For this review, take the finished solid that the model builds, in its own axes (mm). Round coordinates to 2 decimals unless told otherwise and drop trailing zeros. Write each loop counter-clockwise with the first axis right and the second up, starting at its lowest first coordinate (ties: lowest second). Pieces come first, ordered by that corner, then holes.
Autodesk Inventor part; units mm, degrees
ref_plane "YZ Plane" through (0, 0, 0) normal (1, 0, 0) x (0, 1, 0)
ref_plane "XZ Plane" through (0, 0, 0) normal (0, 1, 0) x (-1, 0, 0)
ref_plane "XY Plane" through (0, 0, 0) normal (0, 0, 1) x (1, 0, 0)
sketch "Sketch1" plane through (0, 0, 0) normal (0, 1, 0) x (-1, 0, 0)
  line L0 (0.3129, 0) -> (0.3129, 5)
  line L1 (3.3129, 5) -> (3.3129, 0)
  arc A0 (3.3129, 5) -> (0.3129, 5) centre (1.8129, 5) ccw
  arc A1 (0.3129, 0) -> (3.3129, 0) centre (1.8129, 0) ccw
  point P0 (0, 0)
  dimension "d1" = 5
  dimension "d7" = 3
extrude "Extrusion1" add sketch "Sketch1" along normal blind 3
chamfer "Chamfer1" distance 0.2 angle 45 8 edges at (-0.3129, 3, 2.5) (-1.8129, 3, -1.5) (-1.8129, 3, 6.5) (-3.3129, 3, 2.5) (-0.3129, 0, 2.5) (-1.8129, 0, 6.5) (-3.3129, 0, 2.5) (-1.8129, 0, -1.5)
properties part number "feather_key" material "Stainless Steel"
(1) For pin 1 Ø1.5 at (x, y) = (-3, 1.5) entering from -Z, flat-tipped, find the tip position at first contact; note if it passes through.
Geometry check:
pin 1: stops at z = -1.43
(2) For line 1 along X through (y, z) = (2.85, 3.5); line 2 along Z through (x, y) = (-1.25, 1.55); line 3 along Z through (x, y) = (-1.55, 0.8), list the stretches that pass through material, from the lowest coordinate up.
Geometry check:
line 1: x = -3.26 to -0.36
line 2: z = -1.39 to 6.39
line 3: z = -1.48 to 6.48
(3) We need section A-A, the plane y = 1.55. Give the boundary of the cut face in (x, z), and give its area (3 significant figures).
Geometry check:
outline: (-3.31, 0) arc R1.5 ccw to (-0.31, 0) - (-0.31, 5) arc R1.5 ccw to (-3.31, 5) - close
area: 22.1 mm2
